Autodesk Inventor part; units mm, degrees
ref_plane "YZ Plane" through (0, 0, 0) normal (1, 0, 0) x (0, 1, 0)
ref_plane "XZ Plane" through (0, 0, 0) normal (0, 1, 0) x (-1, 0, 0)
ref_plane "XY Plane" through (0, 0, 0) normal (0, 0, 1) x (1, 0, 0)
sketch "Boceto1" plane through (0, 0, 0) normal (0, 1, 0) x (-1, 0, 0)
  circle A0 centre (0, 0) radius 80
  circle A1 centre (0, 0) radius 77.161
  dimension "d0" = 160
  dimension "d6" = 2.839
extrude "Extrusión3" add sketch "Boceto1" along normal blind 4
extrude "Extrusión4" add sketch "Boceto1" along normal blind 2 contours A1
sketch "Boceto2" plane through (0, 2, 0) normal (0, 1, 0) x (1, 0, 0)
  line L0 (47.5, -3.5651) -> (-47.5, -3.5651)
  line L1 (-47.5, -3.5651) -> (-47.5, 58.4349)
  line L2 (-47.5, 58.4349) -> (47.5, 58.4349)
  line L3 (47.5, 58.4349) -> (47.5, -3.5651)
  line L4 (47.5, -44.1835) -> (-47.5, 44.1835) construction
  line L5 (-47.5, -44.1835) -> (47.5, 44.1835) construction
  line L6 (-48.5, -4.5651) -> (48.5, -4.5651)
  line L7 (48.5, -4.5651) -> (48.5, 59.4349)
  line L8 (48.5, 59.4349) -> (-48.5, 59.4349)
  line L9 (-48.5, 59.4349) -> (-48.5, -4.5651)
  line L10 (-48.5, -9.337) -> (48.5, 54.663) construction
  line L11 (48.5, -45.1835) -> (-48.5, 45.1835) construction
  line L12 (-32.3907, 52.8953) -> (-42.5753, 52.8953)
  line L13 (-42.5753, 52.8953) -> (-42.5753, 45.7711)
  line L14 (-42.5753, 45.7711) -> (-32.3907, 45.7711)
  line L15 (-32.3907, 45.7711) -> (-32.3907, 52.8953)
  point P0 (0, 0)
  dimension "d11" = 95
  dimension "d12" = 62
  dimension "d16" = 1
  dimension "d17" = 1
extrude "Extrusión5" add sketch "Boceto2" along normal blind 12 contours L9 L8 L7 L6
sketch "Boceto4" plane through (-48.5, 2, -59.4349) normal (-1, 0, 0) x (0, 0, 1)
  line L0 (0, 0) -> (0, 12)
  line L1 (0, 12) -> (0, 1.9732)
  line L2 (10, 5.0938) -> (17.4, 5.0938)
  line L3 (17.4, 5.0938) -> (17.4, 7.7938)
  line L4 (17.4, 7.7938) -> (10, 7.7938)
  line L5 (10, 7.7938) -> (10, 5.0938)
  line L6 (10, 5.0938) -> (17.4, 7.7938) construction
  line L7 (17.4, 5.0938) -> (10, 7.7938) construction
  line L8 (9, 4.0938) -> (18.4, 4.0938)
  line L9 (18.4, 4.0938) -> (18.4, 8.7938)
  line L10 (18.4, 8.7938) -> (9, 8.7938)
  line L11 (9, 8.7938) -> (9, 4.0938)
  line L12 (9, 4.0938) -> (18.4, 8.7938) construction
  line L13 (18.4, 4.0938) -> (9, 8.7938) construction
  point P0 (59.4349, -2)
  point P1 (13.7, 6.4438)
  dimension "d22" = 7.4
  dimension "d23" = 2.7
  dimension "d24" = 1
  dimension "d25" = 1
extrude "Extrusión6" cut sketch "Boceto4" against normal blind 14 contours L5 L4 L3 L2
extrude "Extrusión7" add sketch "Boceto4" along normal blind 1
sketch "Boceto6" plane through (0, 2, 0) normal (0, 1, 0) x (1, 0, 0)
  line L0 (-32.4424, -11.0569) -> (36.7172, -11.0569)
  line L1 (36.7172, -11.0569) -> (36.7172, -41.0069)
  line L2 (36.7172, -41.0069) -> (-32.4424, -41.0069)
  line L3 (-32.4424, -41.0069) -> (-32.4424, -11.0569)
  line L4 (-36.4424, -7.0569) -> (40.7172, -7.0569)
  line L5 (40.7172, -7.0569) -> (40.7172, -45.0069)
  line L6 (40.7172, -45.0069) -> (-36.4424, -45.0069)
  line L7 (-36.4424, -45.0069) -> (-36.4424, -7.0569)
  line L8 (36.7172, -7.5569) -> (-32.4424, -7.5569)
  line L9 (-32.4424, -7.5569) -> (-32.4424, -10.5569)
  line L10 (-32.4424, -10.5569) -> (36.7172, -10.5569)
  line L11 (36.7172, -10.5569) -> (36.7172, -7.5569)
  line L12 (36.7172, -44.5069) -> (-32.4424, -44.5069)
  line L13 (-32.4424, -44.5069) -> (-32.4424, -41.5069)
  line L14 (-32.4424, -41.5069) -> (36.7172, -41.5069)
  line L15 (36.7172, -41.5069) -> (36.7172, -44.5069)
  circle A0 centre (38.7172, -9.0569) radius 1
  circle A1 centre (38.7172, -43.0069) radius 1
  circle A2 centre (-34.4424, -9.0569) radius 1
  circle A3 centre (-34.4424, -43.0069) radius 1
  point P0 (0, 0)
  dimension "d32" = 4
  dimension "d41" = 3
  dimension "d42" = 0.5
  dimension "d43" = 2
sketch "Boceto7" plane through (0, 2, 0) normal (0, 1, 0) x (1, 0, 0)
  line L0 (-10.16, -47.9931) -> (10.16, -47.9931)
  line L1 (10.16, -47.9931) -> (10.16, -68.3131)
  line L2 (10.16, -68.3131) -> (-10.16, -68.3131)
  line L3 (-10.16, -68.3131) -> (-10.16, -47.9931)
  line L4 (-10.16, -47.9931) -> (10.16, -68.3131) construction
  line L5 (10.16, -47.9931) -> (-10.16, -68.3131) construction
  line L6 (-11.16, -46.9931) -> (11.16, -46.9931)
  line L7 (11.16, -46.9931) -> (11.16, -69.3131)
  line L8 (11.16, -69.3131) -> (-11.16, -69.3131)
  line L9 (-11.16, -69.3131) -> (-11.16, -46.9931)
  line L10 (-11.16, -46.9931) -> (11.16, -69.3131) construction
  line L11 (11.16, -46.9931) -> (-11.16, -69.3131) construction
  point P0 (0, 0)
  point P1 (0, -58.1531)
  dimension "d34" = 20.32
  dimension "d35" = 20.32
  dimension "d36" = 22.32
  dimension "d37" = 22.32
extrude "Extrusión8" add sketch "Boceto7" along normal blind 2
extrude "Extrusión9" add sketch "Boceto6" along normal blind 5
thread "Rosca1"
thread "Rosca2"
thread "Rosca3"
thread "Rosca4"
extrude "Extrusión10" cut sketch "Boceto2" against normal through all contours L15 L14 L13 L12
sketch "Boceto8" plane through (0, 0, 0) normal (0, -1, 0) x (1, 0, 0)
  line L0 (-42.5753, -52.8953) -> (-32.3907, -52.8953)
  line L1 (-32.3907, -52.8953) -> (-32.3907, -45.7711)
  line L2 (-31.3907, -53.8953) -> (-43.5753, -53.8953)
  line L3 (-43.5753, -53.8953) -> (-43.5753, -44.7711)
  line L4 (-43.5753, -44.7711) -> (-31.3907, -44.7711)
  line L5 (-31.3907, -44.7711) -> (-31.3907, -53.8953)
  line L6 (-31.3907, -53.8953) -> (-43.5753, -44.7711) construction
  line L7 (-43.5753, -53.8953) -> (-31.3907, -44.7711) construction
  line L8 (-42.5753, -52.8953) -> (-42.5753, -45.7711)
  line L9 (-42.5753, -52.8953) -> (-32.3907, -52.8953)
  line L10 (-32.3907, -52.8953) -> (-32.3907, -45.7711)
  line L11 (-32.3907, -45.7711) -> (-42.5753, -45.7711)
  line L12 (-42.5753, -45.7711) -> (-42.5753, -52.8953)
  point P0 (0, 0)
  point P1 (-37.483, -49.3332)
  point P2 (-37.483, -52.8953)
  dimension "d56" = 1
  dimension "d57" = 1
extrude "Extrusión11" cut sketch "Boceto8" against normal blind 1
sketch "Boceto9" plane through (0, 2, 0) normal (0, 1, 0) x (1, 0, 0)
  circle A0 centre (0, 0) radius 77.161
  line L0 (77.161, 0) -> (48.5, 0)
  line L1 (48.5, 59.4349) -> (48.5, -4.5651)
  line L2 (57.3305, 20) -> (68.3305, 20)
  line L3 (68.3305, 20) -> (68.3305, -20)
  line L4 (68.3305, -20) -> (57.3305, -20)
  line L5 (57.3305, -20) -> (57.3305, 20)
  line L6 (57.3305, 20) -> (68.3305, -20) construction
  line L7 (68.3305, 20) -> (57.3305, -20) construction
  point P0 (62.8305, 0)
  dimension "d60" = 11
  dimension "d61" = 40
extrude "Extrusión12" add sketch "Boceto9" along normal blind 12 contours L3 L4 L5 L0 | L0 L5 L2 L3
sketch "Boceto11" plane through (57.3305, 2, 20) normal (0, 0, 1) x (1, 0, 0)
  line L0 (11, 0) -> (0, 0)
  line L1 (0, 0) -> (0, 1)
  line L2 (0, 0) -> (0, 12)
  line L3 (0, 1) -> (11, 1)
  line L4 (11, 0) -> (11, 12)
  line L5 (0, 12) -> (11, 12)
  line L6 (0, 12) -> (0.5, 12)
  line L7 (11, 12) -> (10.5, 12)
  line L8 (10.167, 12) -> (0.833, 12)
  line L9 (0, 0) -> (11, 0)
  line L10 (0, 0) -> (0, 12)
  line L11 (11, 12) -> (0, 12)
  line L12 (11, 0) -> (11, 12)
  point P0 (-57.3305, -2)
  dimension "d64" = 1
sketch "Boceto12" plane through (68.3305, 2, -20) normal (0, 0, -1) x (-1, 0, 0)
  arc A0 (0.833, 12) -> (10.167, 12) centre (5.5, 10.2059) ccw
  arc A1 (0.5311, 10.7631) -> (10.167, 12) centre (5.4899, 10.2844) ccw
  line L0 (0.833, 12) -> (10.167, 12)
  line L1 (11, 0) -> (11, 12)
  point P0 (68.3305, -2)
extrude "Extrusión14" cut sketch "Boceto12" against normal blind 39 contours L0 A1 A0
sketch "Boceto13" plane through (0, 2, 0) normal (0, 1, 0) x (1, 0, 0)
  circle A0 centre (-61.3337, 27.7224) radius 1.5
  circle A1 centre (0, 0) radius 77.161
  circle A2 centre (-61.3337, 27.7224) radius 2
  circle A3 centre (-61.3337, -27.7224) radius 1.5
  circle A4 centre (-61.3337, -27.7224) radius 2
  circle A5 centre (61.3337, 27.7224) radius 1.5
  circle A6 centre (61.3337, 27.7224) radius 2
  circle A7 centre (61.3337, -27.7224) radius 2
  circle A8 centre (61.3337, -27.7224) radius 1.5
  line L0 (-61.3337, -27.7224) -> (0, -27.7224)
  line L1 (0, -27.7224) -> (0, 0)
  dimension "d72" = 3
  dimension "d73" = 4
  dimension "d78" = 27.7224
  dimension "d79" = 61.3337
extrude "Extrusión15" add sketch "Boceto13" along normal blind 2 contours A2 | A4 | A6 | A7
extrude "Extrusión16" cut sketch "Boceto13" against normal blind 2 contours A0 | A3 | A5 | A8
properties part number "base"
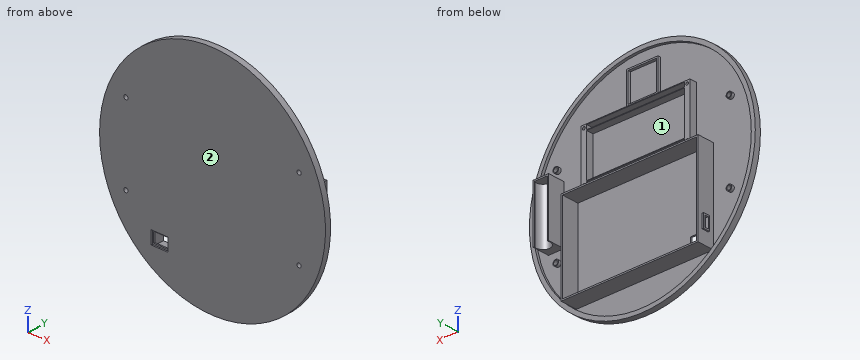
Geometry check sheet. Reference: the model listing, model coordinates, mm. Face numbers are marked on the shaded views. Give positions to 0.01 mm unless a question says otherwise; leave off trailing zeros. Order: outer loops, then holes, each group sorted by start corner. A loop starts at its lowest first (then second) coordinate and runs counter-clockwise, first axis right, second up. Notation, with made-up numbers: (54, 47) - (100, 47) arc R24 cw to (100, 59) - close; hole circle Ø11 at (-12, 35). An arc over 180 degrees is marked (long way). Answer as a JSON object with one key per item and string values.
(1) Cross-section at B-B (z = 0). Record the cut outline in (x, y).
Report:
{"outline": "(-80, 0) - (80, 0) - (80, 4) - (77.16, 4) - (77.16, 2) - (68.33, 2) - (68.33, 14) - (67.5, 14) arc R5 cw to (67.8, 12.76) arc R4.98 cw (long way) to (58.16, 14) - (57.33, 14) - (57.33, 2) - (48.5, 2) - (48.5, 14) - (47.5, 14) - (47.5, 2) - (-47.5, 2) - (-47.5, 14) - (-48.5, 14) - (-48.5, 2) - (-77.16, 2) - (-77.16, 4) - (-80, 4) - close"}
(2) Draft check along X on the marked faces 1 and 2. Enter one of: released by +X, released by -X, zero draft, split by the parting line, or undercut.
Report:
{"face 1": "undercut", "face 2": "zero draft"}
(3) Cross-section at A-A (x = 52). Record the cut outline in (y, z).
Report:
{"outline": "(0, -60.79) - (4, -60.79) - (4, -57.01) - (2, -57.01) - (2, 57.01) - (4, 57.01) - (4, 60.79) - (0, 60.79) - close"}
(4) Depth check by flat-ended pin: pin 1 Ø5 at (y, z) = (2, 36) entering from -X; pin 2 Ø1 at (y, z) = (10, 9) entering from -X; pin 3 Ø0.8 at (x, y) = (-38, 1.5) entering from -Z; pin 4 Ø3 at (x, z) = (54, 11.5) entering from -Y. Enter the tip coordinate at first touch or a pass-through.
Report:
{"pin 1": "x = -72.65", "pin 2": "x = 57.33", "pin 3": "z = -70.61", "pin 4": "y = 0"}
(5) Cross-section at C-C (x = -54.5). Record the cut outline in (y, z), then the cut area to 3 significant figures.
Report:
{"outline": "(0, -58.56) - (4, -58.56) - (4, -54.62) - (2, -54.62) - (2, 54.62) - (4, 54.62) - (4, 58.56) - (0, 58.56) - close", "area": "250 mm^2"}
(6) Cross-section at D-D (z = -34). Record the cut outline in (x, y).
Report:
{"outline": "(-72.42, 0) - (72.42, 0) - (72.42, 4) - (69.27, 4) - (69.27, 2) - (48.5, 2) - (48.5, 14) - (47.5, 14) - (47.5, 2) - (-47.5, 2) - (-47.5, 14) - (-48.5, 14) - (-48.5, 2) - (-69.27, 2) - (-69.27, 4) - (-72.42, 4) - close"}
(7) Material ranges on line 1 (X direction, y = 6, z = -2.5); line 2 (Z direction, x = 33, y = 5.5); line 3 (Z direction, x = 26.5, y = 12), recorded low to high.
Report:
{"line 1": "-48.5 to -47.5, 47.5 to 48.5, 57.33 to 68.33", "line 2": "-59.43 to -58.43, 3.57 to 4.57, 7.06 to 7.56, 10.56 to 11.06, 41.01 to 41.51, 44.51 to 45.01", "line 3": "-59.43 to -58.43, 3.57 to 4.57"}
